Drawing for the job (mm, zero at the part's lowest x, y, z). Give positions to 0.01 mm unless a question says otherwise; leave off trailing zeros. Write each loop counter-clockwise with the first axis right and the second up, starting at its lowest first coordinate (ties: lowest second). Pieces come first, ordered by that corner, then holes. Notation, with made-up numbers: M -10,25.25 L 49,25.25 A20 ccw 49,61.25 Z; hole C 20,4.25 d8. An arc over 180 degrees is marked long. Answer as a JSON object with one key per item and string values. Group by question number.
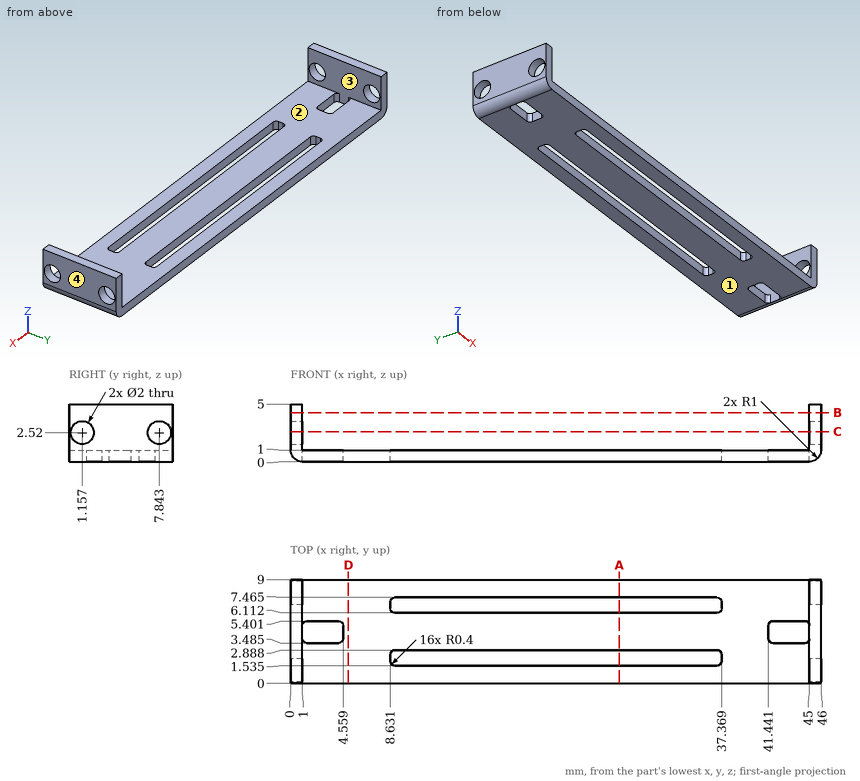
Q1. Slice it at A-A, the plane x = 28.5. Write the cut outline in (y, z) (1 decimal).
Q2. Slice it at D-D, the plane x = 5. Write the cut outline in (y, z).
Q3. Slice it at C-C, the plane z = 2.6. Count the separate pieces of the cut face and the enclosed holes in it.
Q4. Drop flat-ended pins along their axis: P1, Ø2.5, axis at x = 22.5, y = 6, coming from the +Z side; P2, Ø2, axis at x = 22.5, z = 2.5, coming from the -Y side. Give the stop position or say it passes through.
Q5. Two-plate mould, pull along X, no slides. Class the marked faces 1, 2, 3 and 4: +X half, -X half, draft (parallel to the pull), parting line (faces both ways), or undercut.
Q6. Slice it at B-B, the plane z = 4.25. Write the cut outline in (x, y), then the cut area to 3 significant figures.
Q7. Wall check: L1, parallel to X at y = 4.5, z = 0.9 (1 decimal); L2, parallel to X at y = 2, z = 3.7; L3, parallel to Z at x = 41, y = 1.75. Give the ranges that are in metal, low to high.
Solved:
{
 "1": {"outline": "M 0,0 L 1.5,0 L 1.5,1 L 0,1 Z; M 2.9,0 L 6.1,0 L 6.1,1 L 2.9,1 Z; M 7.5,0 L 9,0 L 9,1 L 7.5,1 Z"},
 "2": {"outline": "M 0,0 L 9,0 L 9,1 L 0,1 Z"},
 "3": {"separate pieces": "6", "enclosed holes": "0"},
 "4": {"P1": "stops at z = 1", "P2": "passes through"},
 "5": {"face 1": "draft", "face 2": "undercut", "face 3": "undercut", "face 4": "+X half"},
 "6": {"outline": "M 0,0 L 1,0 L 1,9 L 0,9 Z; M 45,0 L 46,0 L 46,9 L 45,9 Z", "area": "18.0 mm²"},
 "7": {"L1": "x = 0 to 1, 4.6 to 41.4, 45 to 46", "L2": "x = 0 to 1, 45 to 46", "L3": "z = 0 to 1"}
}
